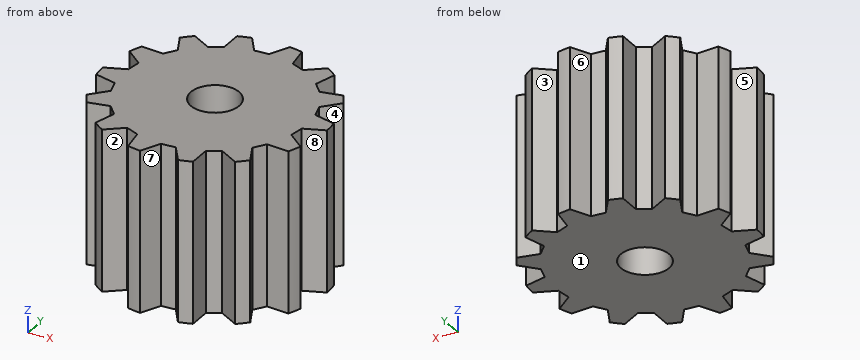
from build123d import *

# Parameters (mm, degrees)
SKETCH1_R           = 1.5
BOSS_EXTRUDE1_DEPTH = 10


with BuildPart() as part:
    # Sketch1 → Boss-Extrude1 (new body)
    with BuildSketch(Plane.XY):
        with BuildLine():
            Line((-2.438077779, 5.096888928), (-2.443359795, 6.452905773))
            ThreePointArc((-2.443359795, 6.452905773), (-2.051006224, 6.588123668), (-1.65123331, 6.699509576))
            Line((-1.65123331, 6.699509576), (-0.861593933, 5.583919403))
            Line((-0.861593933, 5.583919403), (0.01482505, 5.64998055))
            Line((0.01482505, 5.64998055), (0.598419776, 6.874001293))
            ThreePointArc((0.598419776, 6.874001293), (1.010586975, 6.825592573), (1.419098459, 6.752492841))
            Line((1.419098459, 6.752492841), (1.646502519, 5.40476914))
            Line((1.646502519, 5.40476914), (2.464791596, 5.084024232))
            Line((2.464791596, 5.084024232), (3.521674972, 5.933616552))
            ThreePointArc((3.521674972, 5.933616552), (3.87202103, 5.711169157), (4.208360374, 5.468062084))
            Line((4.208360374, 5.468062084), (3.828488954, 4.155138064))
            Line((3.828488954, 4.155138064), (4.426575937, 3.511114563))
            Line((4.426575937, 3.511114563), (5.747419249, 3.818006283))
            ThreePointArc((5.747419249, 3.818006283), (5.966553832, 3.465578648), (6.164104905, 3.100614571))
            Line((6.164104905, 3.100614571), (5.252196198, 2.082530934))
            Line((5.252196198, 2.082530934), (5.511622626, 1.242785594))
            Line((5.511622626, 1.242785594), (6.834816656, 0.946193044))
            ThreePointArc((6.834816656, 0.946193044), (6.879337474, 0.533587785), (6.898972862, 0.119052315))
            Line((6.898972862, 0.119052315), (5.635641572, -0.402546987))
            Line((5.635641572, -0.402546987), (5.505024858, -1.271692304))
            Line((5.505024858, -1.271692304), (6.568494801, -2.113025331))
            ThreePointArc((6.568494801, -2.113025331), (6.429583959, -2.504086684), (6.267414633, -2.886089711))
            Line((6.267414633, -2.886089711), (4.902879015, -2.80789554))
            Line((4.902879015, -2.80789554), (4.408089402, -3.534295945))
            Line((4.408089402, -3.534295945), (5.001201993, -4.753733125))
            ThreePointArc((5.001201993, -4.753733125), (4.706372487, -5.045796073), (4.394518071, -5.319606275))
            Line((4.394518071, -5.319606275), (3.199041139, -4.657105946))
            Line((3.199041139, -4.657105946), (2.438077779, -5.096888928))
            Line((2.438077779, -5.096888928), (2.443359795, -6.452905773))
            ThreePointArc((2.443359795, -6.452905773), (2.051006224, -6.588123668), (1.65123331, -6.699509576))
            Line((1.65123331, -6.699509576), (0.861593933, -5.583919403))
            Line((0.861593933, -5.583919403), (-0.01482505, -5.64998055))
            Line((-0.01482505, -5.64998055), (-0.598419776, -6.874001293))
            ThreePointArc((-0.598419776, -6.874001293), (-1.010586975, -6.825592573), (-1.419098459, -6.752492841))
            Line((-1.419098459, -6.752492841), (-1.646502519, -5.40476914))
            Line((-1.646502519, -5.40476914), (-2.464791596, -5.084024232))
            Line((-2.464791596, -5.084024232), (-3.521674972, -5.933616552))
            ThreePointArc((-3.521674972, -5.933616552), (-3.87202103, -5.711169157), (-4.208360374, -5.468062084))
            Line((-4.208360374, -5.468062084), (-3.828488954, -4.155138064))
            Line((-3.828488954, -4.155138064), (-4.426575937, -3.511114563))
            Line((-4.426575937, -3.511114563), (-5.747419249, -3.818006283))
            ThreePointArc((-5.747419249, -3.818006283), (-5.966553832, -3.465578648), (-6.164104905, -3.100614571))
            Line((-6.164104905, -3.100614571), (-5.252196198, -2.082530934))
            Line((-5.252196198, -2.082530934), (-5.511622626, -1.242785594))
            Line((-5.511622626, -1.242785594), (-6.834816656, -0.946193044))
            ThreePointArc((-6.834816656, -0.946193044), (-6.879337474, -0.533587785), (-6.898972862, -0.119052315))
            Line((-6.898972862, -0.119052315), (-5.635641572, 0.402546987))
            Line((-5.635641572, 0.402546987), (-5.505024858, 1.271692304))
            Line((-5.505024858, 1.271692304), (-6.568494801, 2.113025331))
            ThreePointArc((-6.568494801, 2.113025331), (-6.429583959, 2.504086684), (-6.267414633, 2.886089711))
            Line((-6.267414633, 2.886089711), (-4.902879015, 2.80789554))
            Line((-4.902879015, 2.80789554), (-4.408089402, 3.534295945))
            Line((-4.408089402, 3.534295945), (-5.001201993, 4.753733125))
            ThreePointArc((-5.001201993, 4.753733125), (-4.706372487, 5.045796073), (-4.394518071, 5.319606275))
            Line((-4.394518071, 5.319606275), (-3.199041139, 4.657105946))
            Line((-3.199041139, 4.657105946), (-2.438077779, 5.096888928))
        make_face()
        Circle(SKETCH1_R, mode=Mode.SUBTRACT)
    extrude(amount=BOSS_EXTRUDE1_DEPTH)


solid = part.part
Can you work these out from the model? Positions are in its coordinate system, mm. Face numbers are marked on the shaded views. A direction names the side the tool comes from. Coordinates: 2 decimals unless noted, no trailing zeros. Write each question's results on one line, items separated by ' | '. Start each with the question number.
Q1. On a 3-axis mill with a long thin cutter (end or side, diameter ignored), from which of +Z, -Z, +X, -X, +Y, -Y can I reach the whole of each face in a straight line? I mean the marked faces 5, 6, 7 and 8. Say none if no direction works.
Q2. We'd pull the mould along Y, two halves only. Please class the marked faces 1, 2, 3 and 4: +Y half, -Y half, draft (parallel to the pull), parting line (faces both ways), or undercut.
Q3. If I drill on probe 1 along Y at (x, z) = (-1.25, 6.5); probe 2 along X at (y, z) = (0.75, 6); probe 3 along Y at (x, z) = (-4.75, 6.5), over which ranges is the centre line in solid material (lowest first)?
Q4. I'm going to push flat-ended pins straight in: pin 1 (1 mm diameter, centred on y = 2.5, z = 3, fed in from -X); pin 2 (6 mm diameter, centred on y = 4.5, z = 4, fed in from +X). Where does each tip first touch, or does it pass through?
Taken from the geometry:
1) face 5: +Z, -Z, -X | face 6: +Z, -Z, +Y | face 7: +Z, -Z, -Y | face 8: +Z, -Z, +X
2) face 1: draft | face 2: -Y half | face 3: +Y half | face 4: undercut
3) probe 1: y = -6.79 to -0.83, 0.83 to 6.13 | probe 2: x = -5.58 to -1.3, 1.3 to 6.86 | probe 3: y = -3.59 to 3.03, 4.24 to 5
4) pin 1: stops at x = -6.57 | pin 2: stops at x = 6.16
